from build123d import *

# Parameters (mm, degrees)
F0_R     = 15
F1_DEPTH = 2
F2_R     = 13.45
F3_DEPTH = 5
F4_R     = 0.5
F6_DEPTH = 0.5
F7_R     = 0.1
F8_R     = 11.95
F9_DEPTH = 5


with BuildPart() as f1:
    # F0 (on Top) → F1 (new body)
    with BuildSketch(Plane.XY):
        Circle(F0_R)
    extrude(amount=F1_DEPTH)

    # F2 (on face) → F3 (join)
    with BuildSketch(Plane.XY.offset(2)):
        Circle(F2_R)
    extrude(amount=F3_DEPTH)

    # F4
    f4_edges = [f1.edges().sort_by_distance(p)[0] for p in [
        (-15, 0, 2),
        (-13.45, 0, 7),
        (-15, 0, 0),
    ]]
    fillet(f4_edges, radius=F4_R)

    # F5 (on face) → F6 (join)
    with BuildSketch(Plane(origin=(0, 0, 0), x_dir=(1, 0, 0), z_dir=(0, 0, -1))):
        Polygon((-6.25, -4.082904), (-0.25, -0.618802), (-0.25, 4), (-6.25, 0.535898), align=None)
        Polygon((0.25, 4), (0.25, -0.618802), (4.25, -2.928203), (4.25, 1.690599), align=None)
        Polygon((4, -3.072541), (0, -0.76314), (-6, -4.227241), (-2, -6.536642), align=None)
    extrude(amount=F6_DEPTH)

    # F7
    f7_edges = [f1.edges().sort_by_distance(p)[0] for p in [
        (2.25, 1.773503, -0.5),
        (2.25, -2.845299, -0.5),
        (4.25, 0.618802, -0.5),
        (0.25, -1.690599, -0.5),
        (-0.25, -1.690599, -0.5),
        (-3, 2.495191, -0.5),
        (2, 1.91784, -0.5),
        (1, 4.804592, -0.5),
        (-4, 5.381942, -0.5),
        (-3.25, 2.350853, -0.5),
        (-6.25, 1.773503, -0.5),
        (-3.25, -2.267949, -0.5),
    ]]
    fillet(f7_edges, radius=F7_R)

    # F8 (on face) → F9 (cut)
    with BuildSketch(Plane.XY.offset(7)):
        Circle(F8_R)
    extrude(amount=-F9_DEPTH, mode=Mode.SUBTRACT)


solid = f1.part
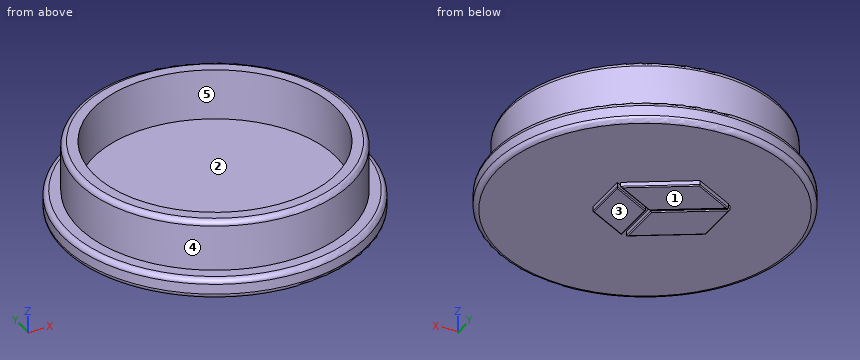
Here's how the part is built. I have some questions about the finished solid (model axes, mm). Face numbers are marked on the shaded views. A direction names the side the tool comes from. Coordinates: 2 decimals unless noted, no trailing zeros. Order: outer loops, then holes, each group sorted by start corner. A loop starts at its lowest first (then second) coordinate and runs counter-clockwise, first axis right, second up. Notation, with made-up numbers: (24.5, -31) - (43.5, -31) arc R14 ccw to (43.5, -11) - close; hole circle Ø6 at (86, -5). An arc over 180 degrees is marked (long way). Use CSV: the item, a comma, the result in double quotes. Start each with the question number.
1. For the marked faces 1 and 2, which set-ups out of +Z, -Z, +X, -X, +Y, -Y let a thin tool reach every point of the face, with its end or its side?
2. Suppose I cut it at B-B on z = 5.5. List the corners of the cut face in (x, y) for me.
3. Please list where these lines run through material, in increasing order: line 1 (Y direction, x = 0, z = 5.85); line 2 (Y direction, x = -10, z = 4.75); line 3 (Z direction, x = -11, y = 5.75). Write a range as from..to.
4. I'm going to push flat-ended pins straight in: pin 1 (5 mm diameter, centred on x = -3.5, y = -10.5, fed in from -Z); pin 2 (4 mm diameter, centred on x = -9.5, z = 4.5, fed in from -Y); pin 3 (7 mm diameter, centred on x = -5.5, y = 5.5, fed in from +Z). Where does each tip first touch, or does it pass through?
5. If we mould it in two halves opening along X, with no side actions, what happens to the marked faces 3, 4 and 5? For each: +X half, -X half, draft (parallel to the pull), parting line (faces both ways), or undercut.
Output:
1,face 1,"-Z, +X, -X, +Y, -Y"
1,face 2,"+Z"
2,outline,"circle Ø26.9 at (0, 0); hole circle Ø23.9 at (0, 0)"
3,line 1,"y = -13.45..-11.95, 11.95..13.45"
3,line 2,"y = -8.99..-6.54, 6.54..8.99"
3,line 3,"z = 0..7"
4,pin 1,"stops at z = 0"
4,pin 2,"stops at y = -11.16"
4,pin 3,"stops at z = 2"
5,face 3,"draft"
5,face 4,"parting line"
5,face 5,"undercut"
